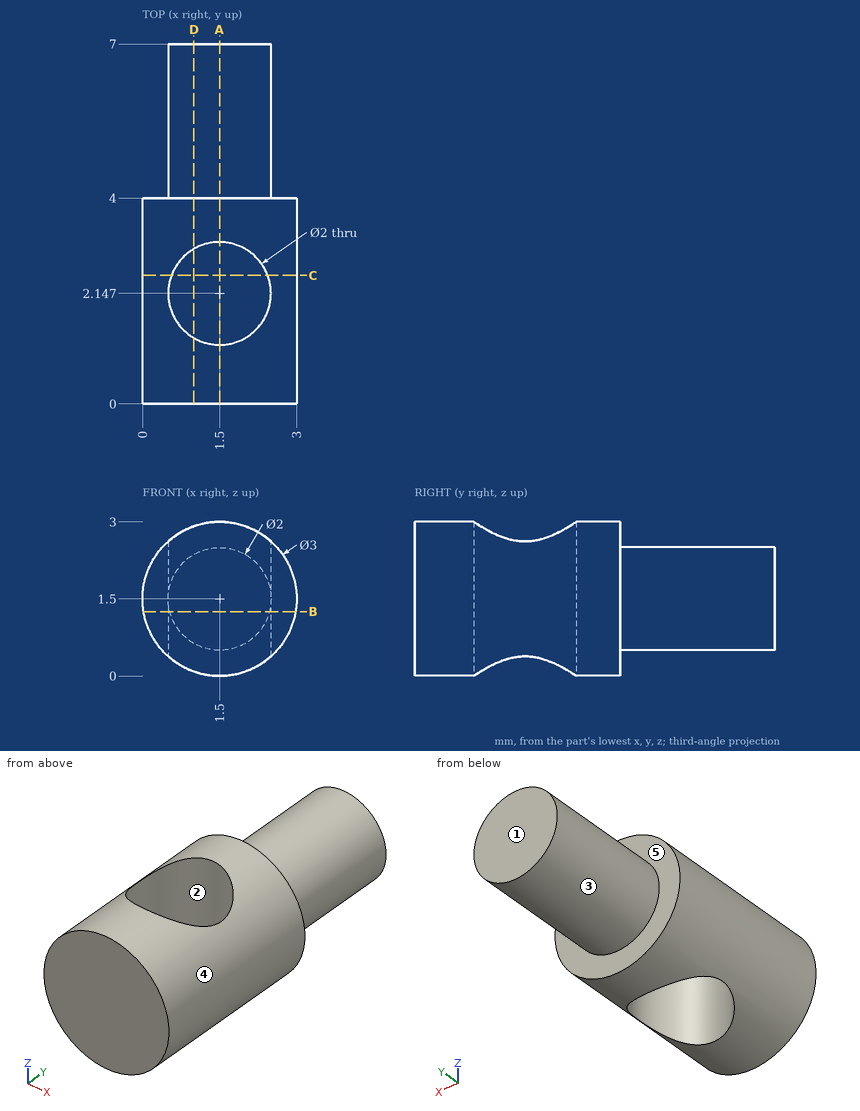
Print and shaded views of the part. All mm, measured from the part's lowest x, y and z. A direction names the side the tool comes from. Give positions to 0.01 mm unless a question says otherwise; leave off trailing zeros. Loops run counter-clockwise (first coordinate to the right, second up) from the corner with the lowest first, then second, coordinate; pieces in that order, holes last. Notation, with made-up numbers: (84, 2.5) -> (91, 2.5) arc R8 ccw to (91, 12.5) -> close; hole circle Ø3 at (85, 41.25). An arc over 180 degrees is marked (long way). Answer in a Markdown table with one row per item.
Item 1: Tool access for the marked faces 4 and 5: list every direction of +Z, -Z, +X, -X, +Y, -Y with a clear straight run to the whole face (end or side of a thin tool).
Findings below:
| item | result |
|---|---|
| face 4 | +Y, -Y |
| face 5 | +Y |
Item 2: Mould opens along X. For the marked faces 1, 2 and 3 say: pulls with the +X half, pulls with the -X half, needs draft (parallel to the pull), parting line crosses it, or undercut.
Findings below:
| item | result |
|---|---|
| face 1 | needs draft |
| face 2 | undercut |
| face 3 | parting line crosses it |
Item 3: Slice it at D-D on x = 1. Write the cut outline in (y, z) (1 decimal).
Findings below:
| item | result |
|---|---|
| outline | (0, 0.1) -> (1.3, 0.1) -> (1.3, 2.9) -> (0, 2.9) -> close; (3, 0.1) -> (4, 0.1) -> (4, 0.6) -> (7, 0.6) -> (7, 2.4) -> (4, 2.4) -> (4, 2.9) -> (3, 2.9) -> close |
Item 4: Probe line 1 along Y through (x, z) = (1.5, 0.7); line 2 along Y through (x, z) = (1.45, 2.75) (1 decimal); line 3 along X through (y, z) = (2.5, 1.95) (1 decimal). List the from-to ranges inside material, lowest first. Write a range as [from, to].
Findings below:
| item | result |
|---|---|
| line 1 | y = [0, 1.15], [3.15, 7] |
| line 2 | y = [0, 1.1], [3.1, 4] |
| line 3 | x = [0.1, 0.6], [2.4, 2.9] |
Item 5: Slice it at A-A on x = 1.5. Write the cut outline in (y, z), plus the area to 3 significant figures.
Findings below:
| item | result |
|---|---|
| outline | (0, 0) -> (1.15, 0) -> (1.15, 3) -> (0, 3) -> close; (3.15, 0) -> (4, 0) -> (4, 0.5) -> (7, 0.5) -> (7, 2.5) -> (4, 2.5) -> (4, 3) -> (3.15, 3) -> close |
| area | 12.0 mm² |
Item 6: Slice it at C-C on y = 2.5. Write the cut outline in (x, z) (1 decimal).
Findings below:
| item | result |
|---|---|
| outline | (0.6, 0.3) -> (0.6, 2.7) arc R1.5 ccw to start; (2.4, 0.3) arc R1.5 ccw to (2.4, 2.7) -> close |
Item 7: Slice it at B-B on z = 1.25. Write the cut outline in (x, y).
Findings below:
| item | result |
|---|---|
| outline | (0.02, 0) -> (2.98, 0) -> (2.98, 4) -> (2.47, 4) -> (2.47, 7) -> (0.53, 7) -> (0.53, 4) -> (0.02, 4) -> close; hole circle Ø2 at (1.5, 2.15) |
Item 8: Flat gauge pin, fed straight in: P1, Ø1, axis at x = 1.5, y = 2, coming from the -Z side. Where does the tip first touch, or does it go through?
Findings below:
| item | result |
|---|---|
| P1 | passes through |
